For this review, use the dimensioned drawing (mm, ordinates from the lowest corner) and the shaded views. A direction names the side the tool comes from. Round coordinates to 2 decimals unless told otherwise and drop trailing zeros. Order: outer loops, then holes, each group sorted by start corner. A loop starts at its lowest first (then second) coordinate and runs counter-clockwise, first axis right, second up. Notation, with made-up numbers: (71, 29) -> (124, 29) arc R24 cw to (124, 47) -> close; hole circle Ø11 at (11, 54). An arc over 180 degrees is marked (long way). Answer in a Markdown table with one row per item.
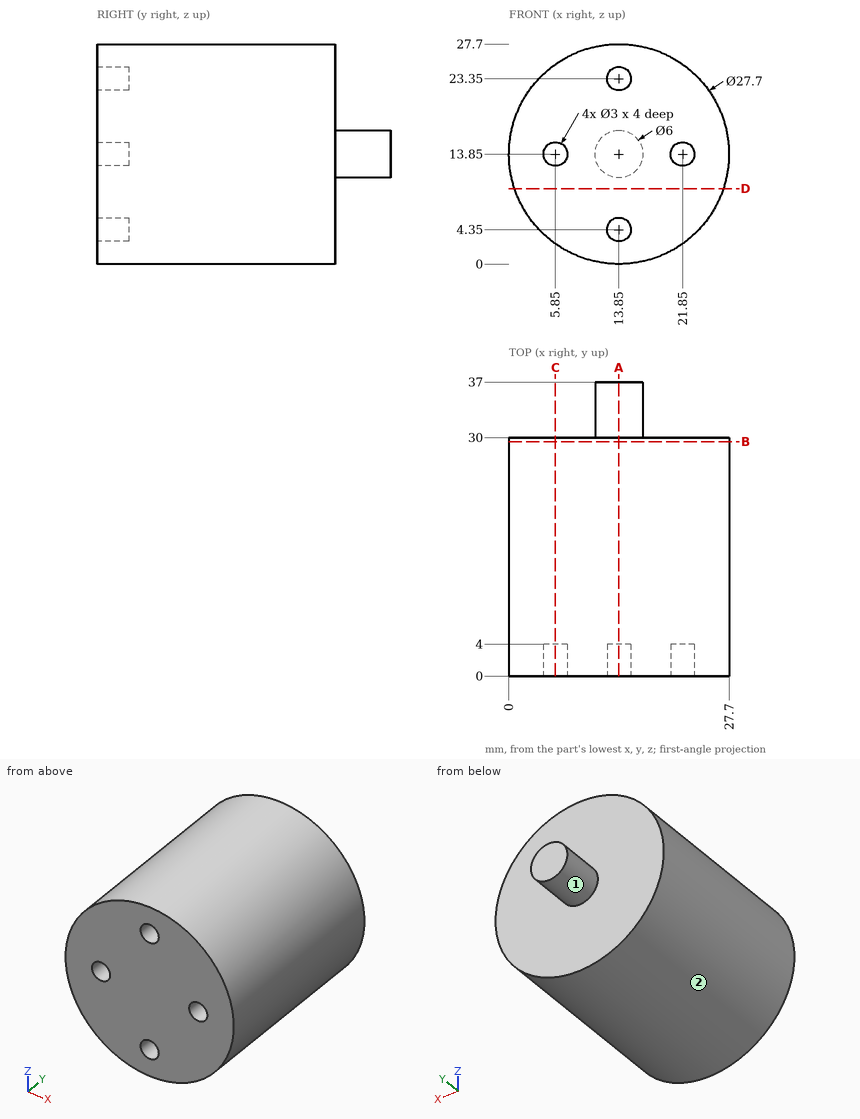
Q1. Take a section at C-C, the plane x = 5.85. Write out the cut boundary in (y, z).
Answer key:
| item | result |
|---|---|
| outline | (0, 2.54) -> (30, 2.54) -> (30, 25.16) -> (0, 25.16) -> (0, 15.35) -> (4, 15.35) -> (4, 12.35) -> (0, 12.35) -> close |
Q2. Tool access review of the marked faces 1 and 2: name each direction out of +Z, -Z, +X, -X, +Y, -Y from which nothing blocks a thin tool from reaching the whole face with its end or side.
Answer key:
| item | result |
|---|---|
| face 1 | +Y |
| face 2 | +Y, -Y |
Q3. Take a section at D-D, the plane z = 9.5. Write out the cut boundary in (x, y).
Answer key:
| item | result |
|---|---|
| outline | (0.7, 0) -> (27, 0) -> (27, 30) -> (0.7, 30) -> close |
Q4. Take a section at B-B, the plane y = 29.5. Write out the cut boundary in (x, z), then the cut area to 3 significant figures.
Answer key:
| item | result |
|---|---|
| outline | circle Ø27.7 at (13.85, 13.85) |
| area | 603 mm^2 |
Q5. Clearance check with flat-ended pins moving along their axes: pin 1 Ø5 at (y, z) = (6.5, 9.5) entering from -X; pin 2 Ø8 at (y, z) = (25.5, 19) entering from -X; pin 3 Ø2.5 at (x, z) = (21.85, 13.85) entering from +Y. State where each tip first meets the part, or that it passes through.
Answer key:
| item | result |
|---|---|
| pin 1 | stops at x = 0.12 |
| pin 2 | stops at x = 0.05 |
| pin 3 | stops at y = 30 |
Q6. Take a section at A-A, the plane x = 13.85. Write out the cut boundary in (y, z).
Answer key:
| item | result |
|---|---|
| outline | (0, 0) -> (30, 0) -> (30, 10.85) -> (37, 10.85) -> (37, 16.85) -> (30, 16.85) -> (30, 27.7) -> (0, 27.7) -> (0, 24.85) -> (4, 24.85) -> (4, 21.85) -> (0, 21.85) -> (0, 5.85) -> (4, 5.85) -> (4, 2.85) -> (0, 2.85) -> close |
Q7. To check wall thickness, follow probe 1 along X at (y, z) = (1, 13.85); probe 2 along Y at (x, z) = (9.5, 9); probe 3 along X at (y, z) = (1.9, 4.35). State the ranges of each line that lie inside material, in increasing order.
Answer key:
| item | result |
|---|---|
| probe 1 | x = 0 to 4.35, 7.35 to 20.35, 23.35 to 27.7 |
| probe 2 | y = 0 to 30 |
| probe 3 | x = 3.77 to 12.35, 15.35 to 23.93 |
